Geometry: final body of the model. Coordinates: model frame, mm. Coordinates: 2 decimals unless noted, no trailing zeros. Loops run counter-clockwise (first coordinate to the right, second up) from the corner with the lowest first, then second, coordinate; pieces in that order, holes last. Notation, with made-up numbers: (-23, -36.75) -> (-2, -36.75) arc R16 ccw to (-2, -31.75) -> close; hole circle Ø6 at (-38, -9). An arc over 180 degrees is marked (long way). One line per item, written item: value. Start each with the question number.
Item 1: Section query B-B on z = 3.5. Return loops of the section in (x, y) (3 decimals).
Item 2: Section query C-C on y = 0. Return loops of the section in (x, z) (3 decimals).
Item 3: Contact query for flat-ended pins moving along their axis: pin 1 Ø3 at (x, z) = (-27, 1.5) entering from +Y; pin 2 Ø1 at (y, z) = (-9, 1.5) entering from +X; pin 3 Ø3 at (y, z) = (2, 1) entering from -X; pin 4 Ø2.5 at (x, y) = (-38.98, -19.06) entering from -Z (3 decimals). Output: stop coordinate, or through.
Item 4: Section query A-A on x = 0. Return loops of the section in (y, z) (3 decimals), then the cut area to 4 significant figures.
Item 5: Section query D-D on y = -42.5. Return loops of the section in (x, z), then the cut area to 3 significant figures.
Item 6: Ray query, probe 1 along Y at (x, z) = (0, 2.05) (3 decimals); probe 2 along Y at (x, z) = (-38, 3.75); probe 3 along X at (y, z) = (-20, 3.9). Return the intervals inside material, ascending. Write a range as from..to.
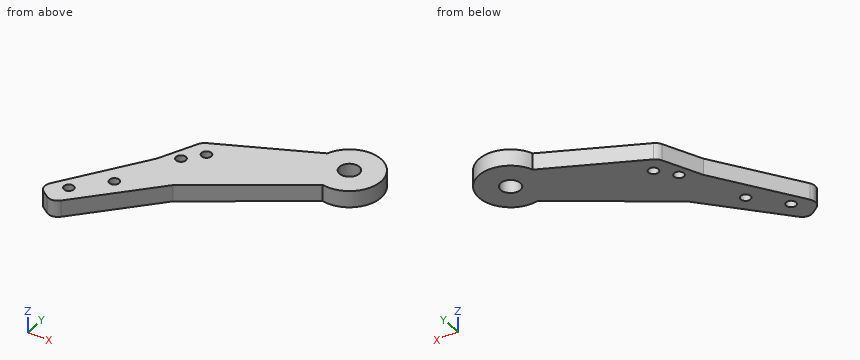
from build123d import *

# Parameters (mm, degrees)
SKETCH_1_R          = 1.5
EXTRUDE_1_DEPTH     = 5
FILLET_1_R          = 3
FILLET_2_R          = 3
FILLET_3_R          = 3
SKETCH_4_R          = 3
CUT_EXTRUDE_1_DEPTH = 82.164250349


with BuildPart() as part:
    # 草图1 → 凸台-拉伸1 (new body)
    with BuildSketch(Plane.XY):
        with BuildLine():
            Line((-2.080891717, -9.376881926), (-34.032481316, -30.39709937))
            Line((-34.032481316, -30.39709937), (-55.995404685, -53.998955167))
            Line((-55.995404685, -53.998955167), (-62.374359774, -49.211848164))
            Line((-62.374359774, -49.211848164), (-44.195107683, -22.4521745))
            Line((-44.195107683, -22.4521745), (-38.494818087, -10.008396594))
            Line((-38.494818087, -10.008396594), (-8.984967737, 3.395052247))
            ThreePointArc((-8.984967737, 3.395052247), (8.44949034, 4.567508949), (-2.080891717, -9.376881926))
        make_face()
        with Locations((-38.975543913, -19.061918057)):
            Circle(SKETCH_1_R, mode=Mode.SUBTRACT)
        with Locations((-34.52729214, -13.94289816)):
            Circle(SKETCH_1_R, mode=Mode.SUBTRACT)
        with Locations((-47.512706739, -37.147272562)):
            Circle(SKETCH_1_R, mode=Mode.SUBTRACT)
        with Locations((-55.63024758, -45.943962561)):
            Circle(SKETCH_1_R, mode=Mode.SUBTRACT)
    extrude(amount=EXTRUDE_1_DEPTH)

    # 圆角1
    fillet_1_edges = [part.edges().sort_by_distance(p)[0] for p in [
        (-55.995404685, -53.998955167, 2.5),
    ]]
    fillet(fillet_1_edges, radius=FILLET_1_R)

    # 圆角2
    fillet_2_edges = [part.edges().sort_by_distance(p)[0] for p in [
        (-62.374359774, -49.211848164, 2.5),
    ]]
    fillet(fillet_2_edges, radius=FILLET_2_R)

    # 圆角3
    fillet_3_edges = [part.edges().sort_by_distance(p)[0] for p in [
        (-38.494818087, -10.008396594, 2.5),
    ]]
    fillet(fillet_3_edges, radius=FILLET_3_R)

    # 草图4 → 切除-拉伸1 (cut, through all)
    with BuildSketch(Plane.XY.offset(5)):
        Circle(SKETCH_4_R)
    extrude(amount=-CUT_EXTRUDE_1_DEPTH, mode=Mode.SUBTRACT)


solid = part.part
Reply:
1. outline: (-60.766, -46.844) arc R3 ccw to (-60.085, -50.93) -> (-58.154, -52.379) arc R3 ccw to (-54.157, -52.023) -> (-34.032, -30.397) -> (-2.081, -9.377) arc R9.605 ccw (long way) to (-8.985, 3.395) -> (-37.475, -9.545) arc R3 ccw to (-38.961, -11.027) -> (-44.195, -22.452) -> close; hole circle Ø3 at (-55.63, -45.944); hole circle Ø3 at (-47.513, -37.147); hole circle Ø3 at (-38.976, -19.062); hole circle Ø3 at (-34.527, -13.943); hole circle Ø6 at (0, 0)
2. outline: (-16.46, 0) -> (-3, 0) -> (-3, 5) -> (-16.46, 5) -> close; (3, 0) -> (9.605, 0) -> (9.605, 5) -> (3, 5) -> close
3. pin 1: stops at y = -4.11
3. pin 2: stops at x = 4.47
3. pin 3: stops at x = -15.36
3. pin 4: passes through
4. outline: (-9.605, 0) -> (-3, 0) -> (-3, 5) -> (-9.605, 5) -> close; (3, 0) -> (9.605, 0) -> (9.605, 5) -> (3, 5) -> close
4. area: 66.05 mm²
5. outline: (-57.81, 0) -> (-45.29, 0) -> (-45.29, 5) -> (-57.81, 5) -> close
5. area: 62.6 mm²
6. probe 1: y = -9.605..-3, 3..9.605
6. probe 2: y = -34.66..-20.2, -17.92..-9.85
6. probe 3: x = -43.07..-40.15, -37.81..-18.23
